Part model, mm, in its own coordinate system. Face numbers are marked on the shaded views. A direction names the side the tool comes from. Give positions to 0.01 mm unless a question says otherwise; leave off trailing zeros. Write each loop counter-clockwise with the first axis right and the second up, starting at its lowest first coordinate (ties: lowest second). Pieces come first, ordered by that corner, then holes. Notation, with made-up numbers: M -39.75,-14.5 L -19.75,-14.5 A32 cw -19.75,11.5 Z; hole C -31,7.5 d2. An arc over 180 degrees is marked long. Use CSV: the item, a comma, the result in double quotes. Start each with the question number.
Item 1: Cut at B-B (x = 0). List the corners of the cut face in (y, z).
Item 2: Which spindle directions (+Z, -Z, +X, -X, +Y, -Y) get a long thin tool onto all of the face, cutting with end or side? Do the marked faces 5, 6 and 7. Say none if no direction does.
Item 3: Cut at D-D (y = 24). List the corners of the cut face in (x, z).
Item 4: Drill centre lines: line 1 (X direction, y = 0, z = 12); line 2 (X direction, y = -32.5, z = -15.5); line 3 (Y direction, x = -15, z = 25). Where is each one in solid material? Low to high. Write a range as [from, to].
Item 5: Cut at C-C (z = -16.5). List the corners of the cut face in (x, y).
Item 6: Cut at A-A (y = 0). List the corners of the cut face in (x, z), then the cut area to 3 significant figures.
Item 7: Mould opens along X. For the marked faces 1, 2, 3 and 4 say: released by +X, released by -X, zero draft, split by the parting line, or undercut.
Item 8: Pin check, flat tips, straight feed: pin 1 (3 mm diameter, centred on y = 4.5, z = 20.5, fed in from +X); pin 2 (8 mm diameter, centred on y = -32, z = -14.5, fed in from -X); pin 3 (2.5 mm diameter, centred on x = 6, y = 31.5, fed in from -Z). Stop position of each tip, or through.
from build123d import *

# Parameters (mm, degrees)
BOSS_EXTRUDE1_DEPTH      = 30
SKETCH2_R                = 4.091242679
BOSS_EXTRUDE2_DEPTH      = 15
SKETCH3_W                = 20
SKETCH3_H                = 12.982921918
BOSS_EXTRUDE3_DEPTH      = 20
BOSS_EXTRUDE5_DEPTH      = 20
BOSS_EXTRUDE5_DEPTH_BACK = 20
SKETCH5_R                = 2.5
SKETCH6_R                = 5
BOSS_EXTRUDE6_DEPTH      = 5
CUT_EXTRUDE1_DEPTH       = 3
FILLET2_R                = 1


with BuildPart() as part:
    # Sketch1 → Boss-Extrude1 (new, symmetric)
    with BuildSketch(Plane.XY):
        with BuildLine():
            Line((-2.5, 27.888169535), (-2.5, 19.843134833))
            ThreePointArc((-2.5, 19.843134833), (0, -20), (2.5, 19.843134833))
            Line((2.5, 19.843134833), (2.5, 27.888169535))
            ThreePointArc((2.5, 27.888169535), (0, -28), (-2.5, 27.888169535))
        make_face()
    extrude(amount=BOSS_EXTRUDE1_DEPTH, both=True)

    # Sketch2 → Boss-Extrude2 (add, symmetric)
    with BuildSketch(Plane.XY):
        with Locations((6.293533022, 30.722501857)):
            Circle(SKETCH2_R)
        with Locations((-6.293533022, 30.722501857)):
            Circle(SKETCH2_R)
    extrude(amount=BOSS_EXTRUDE2_DEPTH, both=True)

    # Sketch3 → Boss-Extrude3 (add)
    with BuildSketch(Plane.XY):
        with Locations((0, -29.508539041)):
            Rectangle(SKETCH3_W, SKETCH3_H)
    extrude(amount=-BOSS_EXTRUDE3_DEPTH)

    # Sketch5 → Boss-Extrude5 (add, two sides: drawn at the far end of the back side and taken through both)
    with BuildSketch(Plane(origin=(0, 0, 0), x_dir=(0, 0, -1), z_dir=(1, 0, 0)).offset(-BOSS_EXTRUDE5_DEPTH_BACK)):
        with Locations((0, 30.722501857)):
            Circle(SKETCH5_R)
    extrude(amount=BOSS_EXTRUDE5_DEPTH + BOSS_EXTRUDE5_DEPTH_BACK)

    # Sketch6 → Boss-Extrude6 (add)
    with BuildSketch(Plane.ZY.offset(20)):
        with Locations((0, 30.722501857)):
            Circle(SKETCH6_R)
    extrude(amount=-BOSS_EXTRUDE6_DEPTH)

    # Sketch7 → Cut-Extrude1 (cut)
    with BuildSketch(Plane.ZY.offset(20)):
        Polygon((1.58771324, 27.972501857), (3.175426481, 30.722501857), (1.58771324, 33.472501857), (-1.58771324, 33.472501857), (-3.175426481, 30.722501857), (-1.58771324, 27.972501857), align=None)
    extrude(amount=-CUT_EXTRUDE1_DEPTH, mode=Mode.SUBTRACT)

    # Fillet2
    fillet2_edges = [part.edges().sort_by_distance(p)[0] for p in [
        (-20, 30.722501857, -5),
    ]]
    fillet(fillet2_edges, radius=FILLET2_R)


solid = part.part
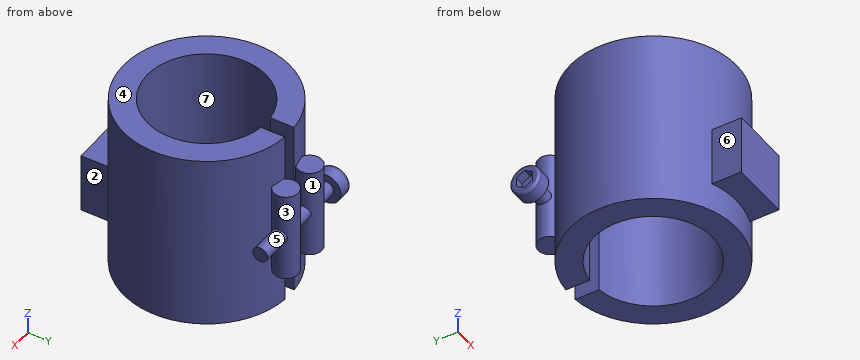
Worked answers:
1,outline,"M -36,-20 L -28,-20 L -28,-30 L -20,-30 L -20,30 L -28,30 L -28,0 L -36,0 Z; C 30.72,0 d5"
2,face 5,"+X"
2,face 6,"+Z, -Z, -X, -Y"
2,face 7,"+Z, -Z"
3,outline,"M -14.42,-30 L -2.5,-30 L -2.5,30 L -14.42,30 Z; M 2.5,-30 L 14.42,-30 L 14.42,30 L 2.5,30 Z"
4,line 1,"x = [-28, -20], [20, 28]"
4,line 2,"x = [-10, 10]"
4,line 3,"y = [-23.64, -13.23], [13.23, 23.64]"
5,outline,"M -10,-36 L 10,-36 L 10,-26.15 A28 ccw 2.5,27.89 L 2.5,19.84 A20 cw long -2.5,19.84 L -2.5,27.89 A28 ccw -10,-26.15 Z"
6,outline,"M -28,-30 L -20,-30 L -20,30 L -28,30 Z; M 20,-30 L 28,-30 L 28,30 L 20,30 Z"
6,area,"960 mm^2"
7,face 1,"undercut"
7,face 2,"released by +X"
7,face 3,"undercut"
7,face 4,"zero draft"
8,pin 1,"stops at x = 27.84"
8,pin 2,"stops at x = -10"
8,pin 3,"stops at z = -15"
